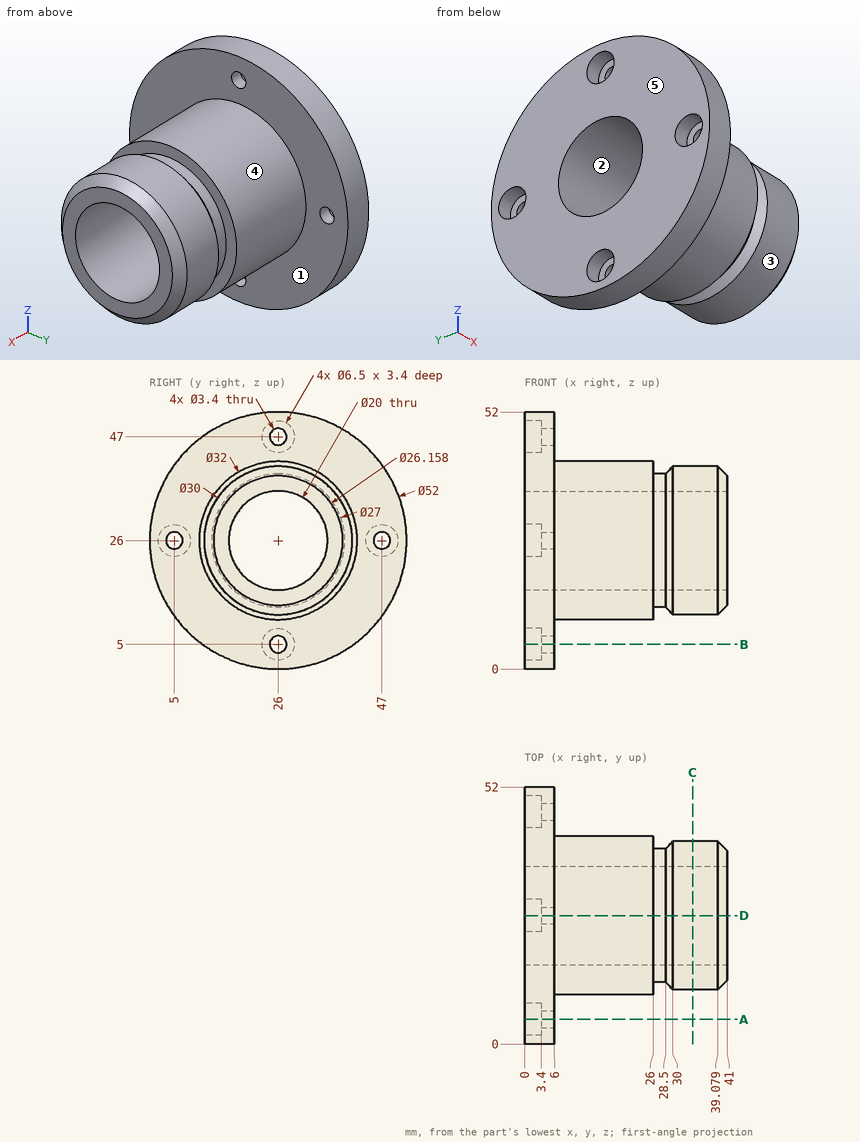
For this review, use the dimensioned drawing (mm, ordinates from the lowest corner) and the shaded views. A direction names the side the tool comes from. Coordinates: 2 decimals unless noted, no trailing zeros. Loops run counter-clockwise (first coordinate to the right, second up) from the corner with the lowest first, then second, coordinate; pieces in that order, holes last. Notation, with made-up numbers: (-32.75, 39.5) -> (0.25, 39.5) arc R33 ccw to (0.25, 73.5) -> close; hole circle Ø7 at (61, 14). An arc over 180 degrees is marked (long way). Return JSON: item names as keys, results as strings. Group by question number.
(1) For pin 1 Ø4 at (y, z) = (38, 40) entering from +X; pin 2 Ø2 at (x, z) = (22, 18.5) entering from -Y; pin 3 Ø4 at (y, z) = (26, 47) entering from -X; pin 4 Ø5 at (y, z) = (33.5, 6.5) entering from -X, all flat-tipped, find the tip position at first contact; note any pin that passes through.
(2) Consider section D-D, the plane y = 26. Count the separate pieces of the cut face and the enclosed holes in it, plus the area to 3 significant figures.
(3) Mouldability with a two-part tool opening along Z and no side actions: class the marked faces 1, 2 and 3 as pulls with the +Z half, pulls with the -Z half, needs draft (parallel to the pull), parting line crosses it, or undercut.
(4) To check wall thickness, follow L1, parallel to Y at x = 5.1, z = 26; L2, parallel to Y at x = 1, z = 26; L3, parallel to X at y = 27, z = 43. State the ranges of each line that lie inside material, in increasing order.
(5) Consider section C-C, the plane x = 34. Give the boundary of the cut face in (y, z).
(6) Consider section A-A, the plane y = 5. Give the boundary of the cut face in (x, z), plus the area to 3 significant figures.
(7) Tool access review of the marked faces 4 and 5: name each direction out of +Z, -Z, +X, -X, +Y, -Y from which nothing blocks a thin tool from reaching the whole face with its end or side.
Results below:
{
 "1": {"pin 1": "stops at x = 6", "pin 2": "stops at y = 11.38", "pin 3": "stops at x = 3.4", "pin 4": "stops at x = 0"},
 "2": {"separate pieces": "4", "enclosed holes": "0", "area": "507 mm2"},
 "3": {"face 1": "needs draft", "face 2": "undercut", "face 3": "parting line crosses it"},
 "4": {"L1": "y = 0 to 3.3, 6.7 to 16, 36 to 45.3, 48.7 to 52", "L2": "y = 0 to 1.75, 8.25 to 16, 36 to 43.75, 50.25 to 52", "L3": "x = 0 to 6"},
 "5": {"outline": "circle Ø30 at (26, 26); hole circle Ø20 at (26, 26)"},
 "6": {"outline": "(0, 10.67) -> (6, 10.67) -> (6, 24.3) -> (3.4, 24.3) -> (3.4, 22.75) -> (0, 22.75) -> close; (0, 29.25) -> (3.4, 29.25) -> (3.4, 27.7) -> (6, 27.7) -> (6, 41.33) -> (0, 41.33) -> close", "area": "153 mm2"},
 "7": {"face 4": "+X", "face 5": "+Z, -Z, -X, +Y, -Y"}
}
